Design review of the part shown in the three views and the two pictorial views. Dimensions are in mm from the part's minimum x, y and z. A direction names the side the tool comes from. Round coordinates to 2 decimals unless told otherwise and drop trailing zeros. Write each loop counter-clockwise with the first axis right and the second up, starting at its lowest first coordinate (ties: lowest second). Pieces come first, ordered by that corner, then holes. Notation, with made-up numbers: (44, 69.25) - (71, 69.25) arc R19 cw to (71, 104.25) - close; hole circle Ø9 at (44, 88). An arc over 180 degrees is marked (long way). Use one line per item in the form item = value.
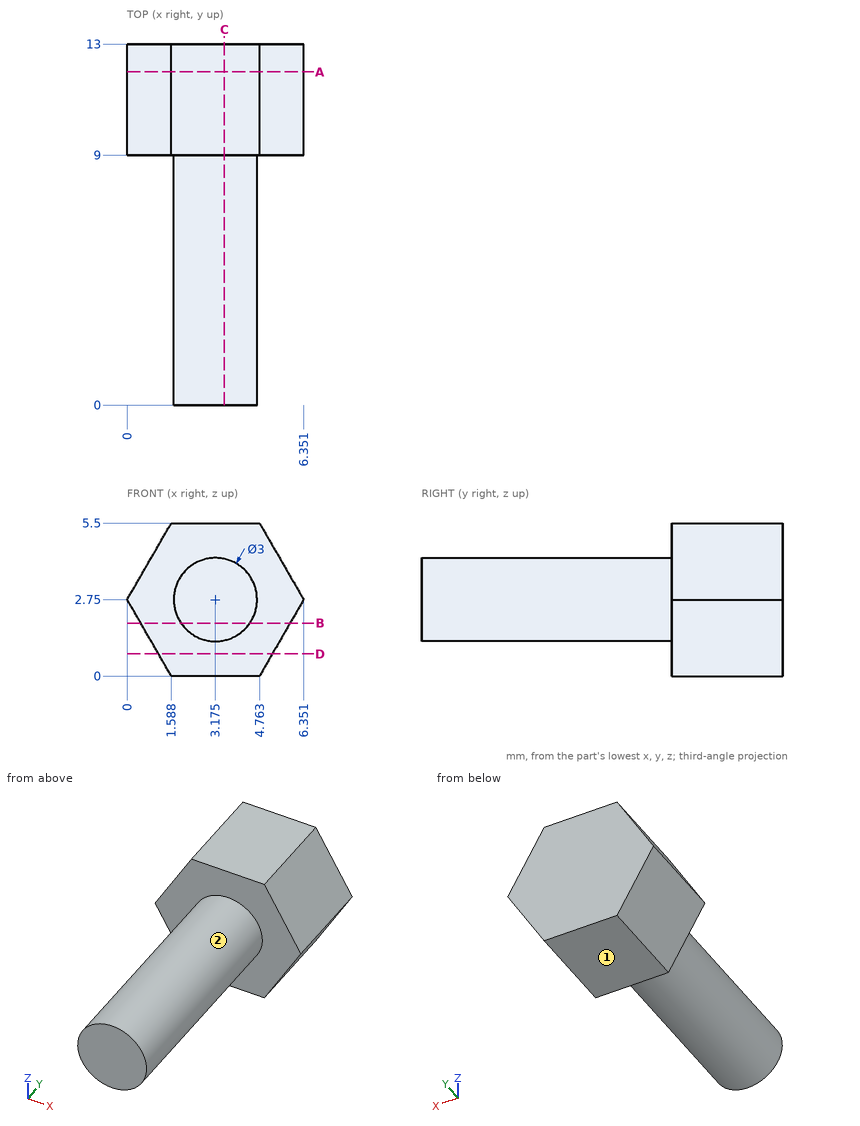
Q1. We need section A-A on y = 12. Write out the cut boundary in (x, z).
Calculated:
outline = (0, 2.75) - (1.59, 0) - (4.76, 0) - (6.35, 2.75) - (4.76, 5.5) - (1.59, 5.5) - close
Q2. We need section B-B on z = 1.9. Write out the cut boundary in (x, y).
Calculated:
outline = (0.49, 9) - (1.94, 9) - (1.94, 0) - (4.41, 0) - (4.41, 9) - (5.86, 9) - (5.86, 13) - (0.49, 13) - close
Q3. We need section C-C on x = 3.5. Write out the cut boundary in (y, z) (1 decimal).
Calculated:
outline = (0, 1.3) - (9, 1.3) - (9, 0) - (13, 0) - (13, 5.5) - (9, 5.5) - (9, 4.2) - (0, 4.2) - close
Q4. We need section D-D on z = 0.8. Write out the cut boundary in (x, y) (1 decimal).
Calculated:
outline = (1.1, 9) - (5.2, 9) - (5.2, 13) - (1.1, 13) - close
Q5. Machinability: for the marked faces 1 and 2, which of the approach directions +Z, -Z, +X, -X, +Y, -Y give a long, thin tool a straight path to every point of the face, cutting with its end or side? Answer none if there is none.
Calculated:
face_1 = -Z, +X, -X, +Y, -Y
face_2 = -Y
Q6. To check wall thickness, follow line 1 along Y through (x, z) = (4.5, 0.55); line 2 along X through (y, z) = (1.5, 1.85) (1 decimal); line 3 along Z through (x, y) = (3.25, 1.75). State the ranges of each line that lie inside material, in increasing order. Write a range as from..to.
Calculated:
line_1 = 9..13
line_2 = 2..4.4
line_3 = 1.25..4.25
